Could you check a few things on this model? Use its own coordinates, in mm. Face numbers are marked on the shaded views. A direction names the side the tool comes from. Round coordinates to 2 decimals unless told otherwise and drop trailing zeros. Loops run counter-clockwise (first coordinate to the right, second up) from the corner with the lowest first, then second, coordinate; pieces in that order, holes last. Notation, with made-up numbers: (-20, 82) - (-5, 82) arc R25 ccw to (-5, 94) - close; hole circle Ø10 at (7, 49.25). An arc over 180 degrees is marked (long way). Use one line per item in the form item = value.
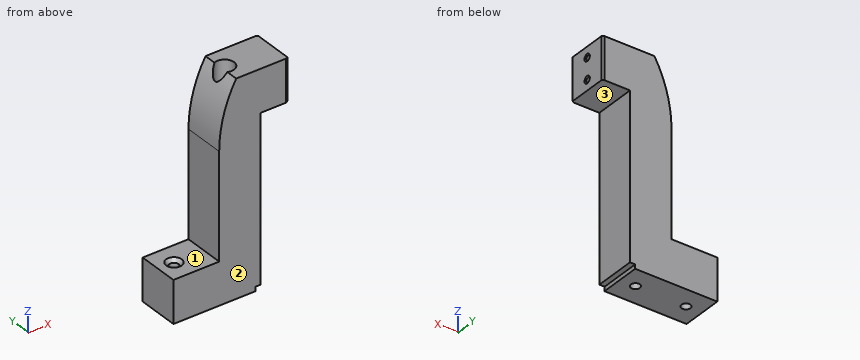
```python
from build123d import *

# Parameters (mm, degrees)
SCHIZZO1_W                             = 39
SCHIZZO1_H                             = 19.7
ESTRUSIONE_ESTRUSIONE1_DEPTH           = 20
FORO_SVASATO_PER_VITE_M4_1_D           = 4.3
FORO_SVASATO_PER_VITE_M4_1_DEPTH       = 20
FORO_SVASATO_PER_VITE_M4_1_CSINK_D     = 7.4
FORO_SVASATO_PER_VITE_M4_1_CSINK_ANGLE = 90
ESTRUSIONE_ESTRUSIONE4_DEPTH           = 80
SCHIZZO7_W                             = 2.463088349
SCHIZZO7_H                             = 19.7
ESTRUSIONE_ESTRUSIONE5_DEPTH           = 18
TAGLIO_ESTRUSIONE2_DEPTH               = 20.7
SCHIZZO17_W                            = 20
SCHIZZO17_H                            = 19.7
ESTRUSIONE_ESTRUSIONE7_DEPTH           = 13.09
SMUSSO1_SIZE                           = 1
SMUSSO1_SIZE2                          = 0.577350269
SMUSSO1_PART_2_SIZE                    = 1
SMUSSO1_PART_2_SIZE2                   = 0.577350269
FORO_SVASATO_PER_VITE_M2_1_D           = 2.4
FORO_SVASATO_PER_VITE_M2_1_DEPTH       = 5
FORO_SVASATO_PER_VITE_M2_1_CSINK_D     = 3.4
FORO_SVASATO_PER_VITE_M2_1_CSINK_ANGLE = 90
FORO_SVASATO_PER_VITE_M2_1_TIP         = 0.721032743


with BuildPart() as part:
    # Schizzo1 → Estrusione-Estrusione1 (new body)
    with BuildSketch(Plane.XY):
        with Locations((19.5, 9.85)):
            Rectangle(SCHIZZO1_W, SCHIZZO1_H)
    extrude(amount=ESTRUSIONE_ESTRUSIONE1_DEPTH)

    # Foro svasato per Vite M4-1
    with Locations(Plane(origin=(7.55, 9.85, 20), x_dir=(1, 0, 0), z_dir=(0, 0, 1))):
        with Locations((0, 0), (24.063088349, 0)):
            CounterSinkHole(FORO_SVASATO_PER_VITE_M4_1_D / 2, FORO_SVASATO_PER_VITE_M4_1_CSINK_D / 2, depth=FORO_SVASATO_PER_VITE_M4_1_DEPTH, counter_sink_angle=FORO_SVASATO_PER_VITE_M4_1_CSINK_ANGLE)

    # Schizzo2 → Estrusione-Estrusione4 (add)
    with BuildSketch(Plane.XY.offset(20)):
        with BuildLine():
            Line((21.763088349, 19.7), (21.763088349, 9.85))
            Line((21.763088349, 9.85), (27.113088349, 9.85))
            ThreePointArc((27.113088349, 9.85), (31.613088349, 14.35), (36.113088349, 9.85))
            Line((36.113088349, 9.85), (39, 9.85))
            Line((39, 9.85), (39, 19.7))
            Line((39, 19.7), (21.763088349, 19.7))
        make_face()
        with BuildLine():
            Line((27.113088349, 9.85), (21.763088349, 9.85))
            Line((21.763088349, 9.85), (21.763088349, 0))
            Line((21.763088349, 0), (39, 0))
            Line((39, 0), (39, 9.85))
            Line((39, 9.85), (36.113088349, 9.85))
            ThreePointArc((36.113088349, 9.85), (31.613088349, 5.35), (27.113088349, 9.85))
        make_face()
        Polygon((39, 9.85), (39, 0), (41.463088349, 0), (41.463088349, 19.7), (39, 19.7), align=None)
    extrude(amount=ESTRUSIONE_ESTRUSIONE4_DEPTH)

    # Schizzo7 → Estrusione-Estrusione5 (add)
    with BuildSketch(Plane(origin=(0, 0, 20), x_dir=(-1, 0, 0), z_dir=(0, 0, -1))):
        with Locations((-40.231544175, 9.85)):
            Rectangle(SCHIZZO7_W, SCHIZZO7_H)
    extrude(amount=ESTRUSIONE_ESTRUSIONE5_DEPTH)

    # Schizzo9 → Taglio-Estrusione2 (cut, through all)
    with BuildSketch(Plane(origin=(0, 19.7, 0), x_dir=(1, 0, 0), z_dir=(0, 1, 0))):
        with BuildLine():
            Line((21.763088349, -70), (21.763088349, -100))
            Line((21.763088349, -100), (29.848264897, -100))
            ThreePointArc((29.848264897, -100), (23.81981051, -85.535202604), (21.763088349, -70))
        make_face()
    extrude(amount=-TAGLIO_ESTRUSIONE2_DEPTH, mode=Mode.SUBTRACT)

    # Schizzo17 → Estrusione-Estrusione7 (add)
    with BuildSketch(Plane(origin=(41.463088349, 0, 0), x_dir=(0, 0, -1), z_dir=(1, 0, 0))):
        with Locations((-90, 9.85)):
            Rectangle(SCHIZZO17_W, SCHIZZO17_H)
    extrude(amount=ESTRUSIONE_ESTRUSIONE7_DEPTH)

    # Smusso1
    smusso1_edges = [part.edges().sort_by_distance(p)[0] for p in [
        (54.553088349, 0, 90),
    ]]
    smusso1_side = [part.faces().sort_by_distance(p)[0] for p in [
        (29.991928904, 0, 46.112902696),
    ]]
    chamfer(smusso1_edges, length=SMUSSO1_SIZE, length2=SMUSSO1_SIZE2, reference=smusso1_side[0])

    # Smusso1 part 2
    smusso1_part_2_edges = [part.edges().sort_by_distance(p)[0] for p in [
        (54.553088349, 19.7, 90),
    ]]
    smusso1_part_2_side = [part.faces().sort_by_distance(p)[0] for p in [
        (29.991928904, 19.7, 46.112902696),
    ]]
    chamfer(smusso1_part_2_edges, length=SMUSSO1_PART_2_SIZE, length2=SMUSSO1_PART_2_SIZE2, reference=smusso1_part_2_side[0])

    # Foro svasato per Vite M2-1
    with Locations(Plane(origin=(54.553088349, 9.85, 95), x_dir=(0, 0, 1), z_dir=(1, 0, 0))):
        with Locations((0, 0), (-10, 0)):
            CounterSinkHole(FORO_SVASATO_PER_VITE_M2_1_D / 2, FORO_SVASATO_PER_VITE_M2_1_CSINK_D / 2, depth=FORO_SVASATO_PER_VITE_M2_1_DEPTH, counter_sink_angle=FORO_SVASATO_PER_VITE_M2_1_CSINK_ANGLE)
            with Locations((0, 0, -(FORO_SVASATO_PER_VITE_M2_1_DEPTH + FORO_SVASATO_PER_VITE_M2_1_TIP / 2))):  # 118° drill point
                Cone(0, FORO_SVASATO_PER_VITE_M2_1_D / 2, FORO_SVASATO_PER_VITE_M2_1_TIP, mode=Mode.SUBTRACT)


solid = part.part
```
1. If we section it at C-C, the plane z = 13: Write out the boundary of the cut face in (x, y).
Solution:
outline = (0, 0) - (41.46, 0) - (41.46, 19.7) - (0, 19.7) - close; hole circle Ø4.3 at (7.55, 9.85); hole circle Ø4.3 at (31.61, 9.85)
2. If we section it at A-A, the plane x = 7.55: Write out the boundary of the cut face in (y, z), plus the area to 3 significant figures.
Solution:
outline = (0, 0) - (7.7, 0) - (7.7, 18.45) - (6.15, 20) - (0, 20) - close; (12, 0) - (19.7, 0) - (19.7, 20) - (13.55, 20) - (12, 18.45) - close
area = 306 mm^2
3. If we section it at D-D, the plane z = 71.5: Write out the boundary of the cut face in (x, y).
Solution:
outline = (21.78, 0) - (41.46, 0) - (41.46, 19.7) - (21.78, 19.7) - close; hole circle Ø9 at (31.61, 9.85)
4. For P1, Ø1.4, axis at y = 9.85, z = 95, coming from the +X side; P2, Ø2, axis at y = 9.85, z = 85, coming from the -X side; P3, Ø1, axis at x = 45.5, y = 14.5, coming from the -Z side, each with a flat end and sliding along its axis, tell me the tip position at first contact or that it passes through.
Solution:
P1 = 49.25
P2 = 23.43
P3 = 80
5. Please list where these lines run through material, in increasing order: line 1 along Z through (x, y) = (51.7, 9.85); line 2 along Y through (x, z) = (51.5, 85); line 3 along X through (y, z) = (9.85, 10).
Solution:
line_1 = 80 to 83.8, 86.2 to 93.8, 96.2 to 100
line_2 = 0 to 8.65, 11.05 to 19.7
line_3 = 0 to 5.4, 9.7 to 29.46, 33.76 to 41.46
6. If we section it at B-B, the plane z = 46: Write out the boundary of the cut face in (x, y), plus the area to 3 significant figures.
Solution:
outline = (21.76, 0) - (41.46, 0) - (41.46, 19.7) - (21.76, 19.7) - close; hole circle Ø9 at (31.61, 9.85)
area = 324 mm^2
7. On a 3-axis mill with a long thin cutter (end or side, diameter ignored), from which of +Z, -Z, +X, -X, +Y, -Y can I reach the whole of each face in a straight line? I mean the marked faces 1, 2 and 3. Say none if no direction works.
Solution:
face_1 = +Z, -X, +Y, -Y
face_2 = +Z, -Z, +X, -X, -Y
face_3 = -Z, +X, +Y, -Y
